For this review, take the finished solid that the model builds, in its own axes (mm). Face numbers are marked on the shaded views. A direction names the side the tool comes from. Give positions to 0.01 mm unless a question says otherwise; leave off trailing zeros. Loops run counter-clockwise (first coordinate to the right, second up) from the corner with the lowest first, then second, coordinate; pieces in that order, holes last.
Autodesk Inventor part; units mm, degrees
ref_plane "Work Plane2" through (21, -90, 18.7376) normal (0, 0, 1) x (1, 0, 0)
ref_plane "Work Plane4" through (25.5777, -4.55, 13.1) normal (0, 0, 1) x (1, 0, 0)
ref_plane "YZ Plane" through (0, 0, 0) normal (1, 0, 0) x (0, 1, 0)
ref_plane "Work Plane1" through (-1.2111, 0.775, 9.6) normal (0, 0, 1) x (0, -1, 0)
sketch "Sketch1" plane through (-1.2111, 0.775, 9.6) normal (0, 0, 1) x (0, -1, 0)
  circle A0 centre (3.575, 28.5389) radius 1.75 construction
  circle A1 centre (-13.125, -18.1803) radius 2 construction
  arc A2 (15.225, -15.8355) -> (15.225, -18.7868) centre (13.875, -17.3111) ccw construction
  line L0 (15.225, -15.8355) -> (15.225, 22.2111) construction
  arc A3 (15.225, 22.2111) -> (-15.225, 22.2111) centre (0, 21.8802) ccw construction
  line L1 (-15.225, 22.2111) -> (-15.225, -22.2111) construction
  line L2 (-15.225, -22.2111) -> (15.225, -22.2111) construction
  line L3 (15.225, -22.2111) -> (15.225, -18.7868) construction
  arc A4 (15.025, 22.209) -> (-15.025, 22.209) centre (0, 21.8802) ccw
  line L4 (15.025, 22.209) -> (15.025, -15.4356)
  arc A5 (15.025, -15.4356) -> (15.025, -19.1866) centre (13.875, -17.3111) ccw
  line L5 (15.025, -19.1866) -> (15.025, -22.0111)
  line L6 (15.025, -22.0111) -> (-14.956, -22.0111)
  arc A6 (-15.025, -18.8048) -> (-15.025, -17.5558) centre (-13.125, -18.1803) ccw construction
  circle A7 centre (3.575, 28.5389) radius 2.25
  arc A8 (-14.9598, -19.0514) -> (-14.9748, -17.3415) centre (-13.125, -18.1803) ccw
  line L7 (-14.956, -22.0111) -> (-14.9598, -19.0514)
  line L8 (-14.9748, -17.3415) -> (-15.025, 22.209)
  point P0 (0.775, 1.2111)
  dimension "d0" = 0.2
  dimension "d1" = 0.5
ref_plane "Work Plane2" through (21, -90, 18.7376) normal (0, 0, 1) x (1, 0, 0)
extrude "Extrusion1" add sketch "Sketch1" along normal blind 10
sketch "Sketch2" plane through (-16.6468, -14.25, 19.6) normal (0, 0, 1) x (1, 0, 0)
  circle A0 centre (16.6468, 14.25) radius 12.3406
  line L0 (4.3062, 14.25) -> (22.8171, 24.9373)
  line L1 (22.8171, 24.9373) -> (22.8171, 3.5627)
  line L2 (22.8171, 3.5627) -> (4.3062, 14.25)
ref_plane "Work Plane3" through (-12.3406, 0, 19.6) normal (-1, 0, 0) x (0, 0, 1)
sketch "Sketch3" plane through (-12.3406, 0, 19.6) normal (-1, 0, 0) x (0, 0, 1)
  line L0 (-0.8319, 0) -> (-10, 0)
  line L1 (-10, 15.8) -> (-10, -14.25)
  circle A0 centre (-1.4284, 0) radius 2.6
  line L2 (1.1716, 0) -> (-4.0284, 0)
  point P0 (-19.6, 0)
  dimension "d4" = 5.2
revolve "Revolution1" cut sketch "Sketch3" angle 360 about axis through (-12.3406, 0, 18.7681) along (0, 0, -1) picked at (-2.9377, -0.2074) contours L2 A0 L0
pattern_circular "Circular Pattern1" count 3 over 360 about axis through (0, 0, 19.6) along (0, 0, 1) of "Revolution1"
ref_plane "Work Plane4" through (25.5777, -4.55, 13.1) normal (0, 0, 1) x (1, 0, 0)
sketch "Sketch5" plane through (-1.2111, 0.775, 19.6) normal (0, 0, 1) x (1, 0, 0)
  circle A0 centre (1.2111, -0.775) radius 16.9061
  circle A1 centre (7.3815, 9.9123) radius 2.1725
  circle A2 centre (7.3815, -11.4623) radius 2.1725
  circle A3 centre (-11.1295, -0.775) radius 2.1725
  circle A4 centre (28.5389, -3.575) radius 2.25
  arc A5 (22.209, -15.025) -> (22.209, 15.025) centre (21.8802, 0) ccw
  line L0 (22.209, 15.025) -> (-17.3415, 14.9748)
  arc A6 (-19.0514, 14.9598) -> (-17.3415, 14.9748) centre (-18.1803, 13.125) ccw
  line L1 (-19.0514, 14.9598) -> (-22.0111, 14.956)
  line L2 (-22.0111, 14.956) -> (-22.0111, -15.025)
  line L3 (-22.0111, -15.025) -> (-19.1866, -15.025)
  arc A7 (-15.4356, -15.025) -> (-19.1866, -15.025) centre (-17.3111, -13.875) ccw
  line L4 (-15.4356, -15.025) -> (22.209, -15.025)
  line L5 (22.209, 15.025) -> (-17.3415, 14.9748)
  line L6 (-15.4356, -15.025) -> (22.209, -15.025)
  point P0 (7.2754, 15.006)
  point P1 (-4.8932, 14.9906)
  point P2 (-7.8858, -15.025)
  point P3 (10.3081, -15.025)
extrude "Extrusion3" cut sketch "Sketch5" against normal up to surface (6.5 mm away) contours A0 L0 A5 L4 | A0 L4 A7 L3 L2 L1 A6 L0
sketch "Sketch6" plane through (-1.2111, 0.775, 13.1) normal (0, 0, 1) x (1, 0, 0)
  circle A0 centre (28.5389, -3.575) radius 2.25
  arc A1 (22.209, -15.025) -> (22.209, 15.025) centre (21.8802, 0) ccw
  line L0 (7.2754, 15.006) -> (22.209, 15.025)
  arc A2 (10.3081, -15.025) -> (7.2754, 15.006) centre (1.2111, -0.775) ccw
  line L1 (22.209, -15.025) -> (10.3081, -15.025)
  arc A3 (-19.0514, 14.9598) -> (-17.3415, 14.9748) centre (-18.1803, 13.125) ccw
  line L2 (-22.0111, 14.956) -> (-19.0514, 14.9598)
  line L3 (-22.0111, -15.025) -> (-22.0111, 14.956)
  line L4 (-19.1866, -15.025) -> (-22.0111, -15.025)
  arc A4 (-15.4356, -15.025) -> (-19.1866, -15.025) centre (-17.3111, -13.875) ccw
  line L5 (-7.8858, -15.025) -> (-15.4356, -15.025)
  arc A5 (-4.8932, 14.9906) -> (-7.8858, -15.025) centre (1.2111, -0.775) ccw
  line L6 (-17.3415, 14.9748) -> (-4.8932, 14.9906)
  circle A6 centre (-18.1803, 13.125) radius 1
  circle A7 centre (-17.3111, -13.875) radius 1
  circle A8 centre (28.5389, -3.575) radius 1
  arc A9 (-19.0514, 14.9598) -> (-17.3415, 14.9748) centre (-18.1803, 13.125) ccw
  line L7 (-17.3415, 14.9748) -> (-19.0514, 14.9598)
  line L8 (-15.4356, -15.025) -> (-19.1866, -15.025)
  point P0 (1.2111, -0.775)
  dimension "d13" = 2
  dimension "d14" = 2
  dimension "d15" = 2
extrude "Extrusion4" add sketch "Sketch6" along normal blind 1 contours A0 | L1 A2 L0 A1 | L7 A3 | A3 L6 A5 L5 A4 L4 L3 L2 | A4 L8
properties part number "03_Insert_Chip_solid"
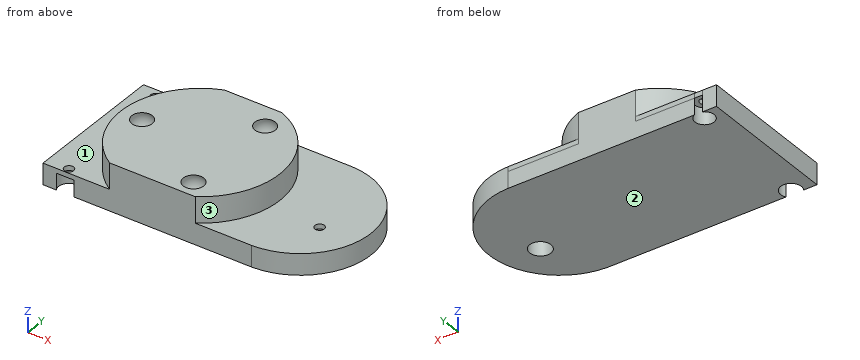
Q1. Consider section C-C on x = -14. Give the boundary of the cut face in (y, z), plus the area to 3 significant figures.
Answers:
outline: (-14.25, 9.6) - (15.76, 9.6) - (15.76, 14.1) - (9.48, 14.1) - (9.48, 19.6) - (1.4, 19.6) arc R2 cw (long way) to (-1.4, 19.6) - (-9.48, 19.6) - (-9.48, 14.1) - (-14.25, 14.1) - close
area: 228 mm2
Q2. For probe 1 along Y at (x, z) = (4.5, 18.5); probe 2 along Y at (x, z) = (25.5, 12); probe 3 along Z at (x, y) = (8.5, -11), list the stretches that pass through material, from the lowest coordinate up.
Answers:
probe 1: y = -14.25 to -12.65, -8.72 to 8.72, 12.65 to 15.78
probe 2: y = -13.46 to -4.11, -1.49 to 15.01
probe 3: z = 9.6 to 17.06, 19.28 to 19.6
Q3. Consider section A-A on y = 13.9. Give the boundary of the cut face in (x, z).
Answers:
outline: (-23.22, 9.6) - (-21.42, 9.6) - (-21.42, 13.1) - (-20.39, 13.1) - (-20.39, 14.1) - (-23.22, 14.1) - close; (-18.39, 13.1) - (-17.36, 13.1) - (-17.36, 9.6) - (27.99, 9.6) - (27.99, 14.1) - (9.62, 14.1) - (9.62, 19.6) - (-9.62, 19.6) - (-9.62, 14.1) - (-18.39, 14.1) - close
Q4. For pin 1 Ø5 at (x, y) = (27.33, -2.8) entering from +Z; pin 2 Ø4 at (y, z) = (-3, 18) entering from +X; pin 3 Ø3 at (x, y) = (27.33, -2.8) entering from -Z, all flat-tipped, find the tip position at first contact; note any pin that passes through.
Answers:
pin 1: stops at z = 14.1
pin 2: stops at x = 16.88
pin 3: stops at z = 13.1
Q5. Consider section D-D on y = -6.5. Give the boundary of the cut face in (x, z).
Answers:
outline: (-23.22, 9.6) - (33.82, 9.6) - (33.82, 14.1) - (15.61, 14.1) - (15.61, 19.6) - (-15.61, 19.6) - (-15.61, 14.1) - (-23.22, 14.1) - close
Q6. Machinability: for the marked faces 1, 2 and 3, which of the approach directions +Z, -Z, +X, -X, +Y, -Y give a long, thin tool a straight path to every point of the face, cutting with its end or side? Answer none if there is none.
Answers:
face 1: +Z, -X
face 2: -Z, +X, -X, +Y, -Y
face 3: +Z, +X
